Drawing for the job (mm, zero at the part's lowest x, y, z). A direction names the side the tool comes from. Give positions to 0.01 mm unless a question says otherwise; leave off trailing zeros. Loops run counter-clockwise (first coordinate to the right, second up) from the corner with the lowest first, then second, coordinate; pieces in that order, holes last. Notation, with made-up numbers: M -6.5,58 L 50.5,58 A15 ccw 50.5,69 Z; hole C 76.5,76.25 d7. An arc over 180 degrees is marked long. Use CSV: the item, a comma, the result in double quotes. Start each with the question number.
(1) Slice it at A-A on z = 4. List the corners of the cut face in (x, y), and give its area (3 significant figures).
(2) Slice it at D-D on y = 2.5. List the corners of the cut face in (x, z), and give its area (3 significant figures).
(3) Slice it at B-B on x = 4. List the corners of the cut face in (y, z).
(4) Tool access for the marked faces 1 and 2: list every direction of +Z, -Z, +X, -X, +Y, -Y with a clear straight run to the whole face (end or side of a thin tool).
(5) Flat gauge pins, fed straight in: P1, Ø2, axis at x = 1, y = 5.5, coming from the +Z side; P2, Ø4, axis at y = 5, z = 1.5, coming from the +X side; P3, Ø4, axis at x = 7, y = 3, coming from the -Z side. Where does each tip first touch, or does it go through?
(6) Slice it at C-C on x = 0.75. List the corners of the cut face in (y, z).
(7) Wall check: line 1 along Y through (x, z) = (0.75, 5.5); line 2 along Z through (x, y) = (4, 3.25); line 3 along Z through (x, y) = (4, 2.5). Give the ranges that are in metal, low to high. Write a range as from..to.
(8) Two-plate mould, pull along Y, no slides. Class the marked faces 3, 4 and 5: pulls with the +Y half, pulls with the -Y half, needs draft (parallel to the pull), parting line crosses it, or undercut.
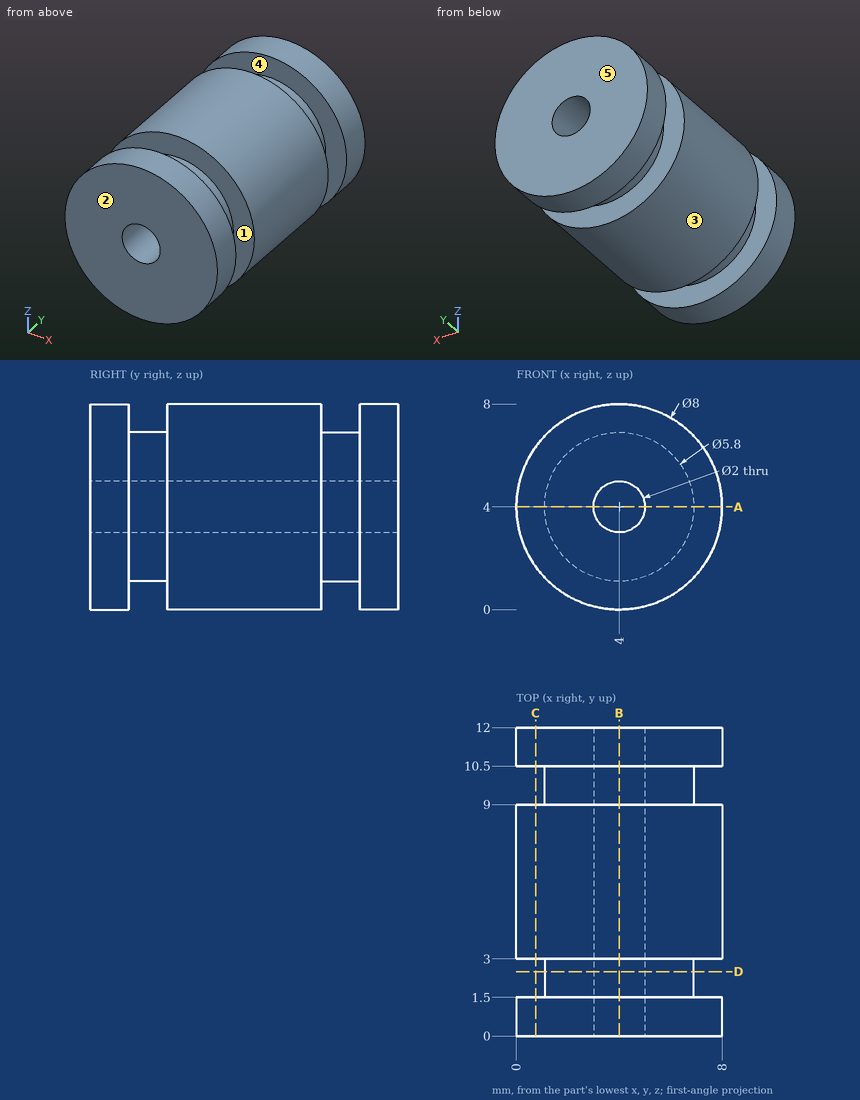
Reply:
1,outline,"M 0,0 L 3,0 L 3,12 L 0,12 L 0,10.5 L 1.1,10.5 L 1.1,9 L 0,9 L 0,3 L 1.1,3 L 1.1,1.5 L 0,1.5 Z; M 5,0 L 8,0 L 8,1.5 L 6.9,1.5 L 6.9,3 L 8,3 L 8,9 L 6.9,9 L 6.9,10.5 L 8,10.5 L 8,12 L 5,12 Z"
1,area,"65.4 mm^2"
2,outline,"C 4,4 d5.8; hole C 4,4 d2"
2,area,"23.3 mm^2"
3,outline,"M 0,0 L 1.5,0 L 1.5,1.1 L 3,1.1 L 3,0 L 9,0 L 9,1.1 L 10.5,1.1 L 10.5,0 L 12,0 L 12,3 L 0,3 Z; M 0,5 L 12,5 L 12,8 L 10.5,8 L 10.5,6.9 L 9,6.9 L 9,8 L 3,8 L 3,6.9 L 1.5,6.9 L 1.5,8 L 0,8 Z"
4,face 1,"none"
4,face 2,"+Z, -Z, +X, -X, -Y"
5,P1,"stops at z = 7.46"
5,P2,"stops at x = 7.97"
5,P3,"stops at z = 0.13"
6,outline,"M 0,1.67 L 1.5,1.67 L 1.5,6.33 L 0,6.33 Z; M 3,1.67 L 9,1.67 L 9,6.33 L 3,6.33 Z; M 10.5,1.67 L 12,1.67 L 12,6.33 L 10.5,6.33 Z"
7,line 1,"y = 0..1.5, 3..9, 10.5..12"
7,line 2,"z = 0..3, 5..8"
7,line 3,"z = 1.1..3, 5..6.9"
8,face 3,"needs draft"
8,face 4,"undercut"
8,face 5,"pulls with the +Y half"
